from build123d import *

# Parameters (mm, degrees)
F0_W     = 90.770632
F0_H     = 82.823328
F1_DEPTH = 25.4
F2_R     = 24.860346
F3_DEPTH = 25.4
F5_DEPTH = 90.771632


with BuildPart() as f1:
    # F0 (on Top) → F1 (new body)
    with BuildSketch(Plane.XY):
        Rectangle(F0_W, F0_H)
    extrude(amount=F1_DEPTH)

    # F2 (on face) → F3 (join)
    with BuildSketch(Plane.XY.offset(25.4)):
        with Locations((5.451556, 0)):
            Circle(F2_R)
    extrude(amount=F3_DEPTH)

    # F4 (on face) → F5 (cut, through all)
    with BuildSketch(Plane.YZ.offset(45.385316)):
        Polygon((24.860346, 50.8), (-24.860346, 50.8), (24.860346, 32.836914), align=None)
    extrude(amount=-F5_DEPTH, mode=Mode.SUBTRACT)


solid = f1.part
Could you check a few things on this model? Use its own coordinates, in mm. A direction names the side the tool comes from. Coordinates: 2 decimals unless noted, no trailing zeros. Write each loop counter-clockwise with the first axis right and the second up, starting at its lowest first coordinate (ties: lowest second). Pieces come first, ordered by that corner, then holes. Notation, with made-up numbers: (-6, 41) - (1, 41) arc R33 cw to (1, 73) - close; hole circle Ø2 at (37, 61.25). An arc over 180 degrees is marked (long way). Put each result on its own line as item: value. Start each with the question number.
Q1. I want a section at D-D on x = 38. Write out the boundary of the cut face in (y, z), plus the area to 3 significant figures.
Q2. I'm going to push flat-ended pins straight in: P1, Ø8, axis at x = -22, y = -30.5, coming from the +Z side; P2, Ø25, axis at x = -2, y = -7.5, coming from the +Z side; P3, Ø6, axis at y = 6.5, z = 30, coming from the -X side. Where does each tip first touch, or does it pass through?
Q3. I want a section at A-A on y = -6.5. Write out the boundary of the cut face in (x, z), plus the area to 3 significant figures.
Q4. Which directions (+Z, -Z, +X, -X, +Y, -Y) give clear straight access to the entire face, cutting with the end or side of a thin tool? Please do faces 1 (the cylindrical face through (0.06, -24.27, 35.1)), 2 (the flat face through (-1, 41.412, 13)).
Q5. I want a section at B-B on x = 3.5. Write out the boundary of the cut face in (y, z), plus the area to 3 significant figures.
Q6. Please list where these lines run through material, in increasing order: L1, parallel to Y at x = 6.5, z = 26.5; L2, parallel to Z at x = 23, y = 23.5; L3, parallel to Z at x = -0.5, y = 2.5.
Q7. I want a section at C-C on z = 30. Write out the boundary of the cut face in (x, y), plus the area to 3 significant figures.
Checks:
1. outline: (-41.41, 0) - (41.41, 0) - (41.41, 25.4) - (-41.41, 25.4) - close
1. area: 2,100 mm²
2. P1: z = 25.4
2. P2: z = 49.04
2. P3: x = -19.16
3. outline: (-45.39, 0) - (45.39, 0) - (45.39, 25.4) - (29.45, 25.4) - (29.45, 44.17) - (-18.54, 44.17) - (-18.54, 25.4) - (-45.39, 25.4) - close
3. area: 3,210 mm²
4. face 1: +Z
4. face 2: +Z, -Z, +X, -X, +Y
5. outline: (-41.41, 0) - (41.41, 0) - (41.41, 25.4) - (24.78, 25.4) - (24.78, 32.86) - (-24.78, 50.77) - (-24.78, 25.4) - (-41.41, 25.4) - close
5. area: 2,920 mm²
6. L1: -24.84 to 24.84
6. L2: 0 to 25.4
6. L3: 0 to 40.92
7. outline: circle Ø49.72 at (5.45, 0)
7. area: 1,940 mm²
